```python
from build123d import *

# Parameters (mm, degrees)
F0_R            = 33
F1_DEPTH        = 2.2
F2_R            = 33
F2_R_2          = 30.8
F3_DEPTH        = 12
F4_R            = 2.2
F5_R            = 2.2
F6_R            = 8
F7_DEPTH        = 2.2
F8_R            = 5.75
F9_DEPTH        = 15.3
F10_W           = 1
F10_H           = 63
F11_DEPTH       = 8
F12_W           = 63
F12_H           = 1
F13_DEPTH       = 8
F15_D           = 0.01
F15_DEPTH       = 2.4
F15_CBORE_D     = 12.2
F15_CBORE_DEPTH = 2.4
F15_TIP         = 0.0030043031


with BuildPart() as f1:
    # F0 (on Top) → F1 (new body)
    with BuildSketch(Plane.XY):
        Circle(F0_R)
    extrude(amount=F1_DEPTH)

    # F2 (on face) → F3 (join)
    with BuildSketch(Plane.XY.offset(2.2)):
        Circle(F2_R)
        Circle(F2_R_2, mode=Mode.SUBTRACT)
    extrude(amount=F3_DEPTH)

    # F4
    f4_edges = [f1.edges().sort_by_distance(p)[0] for p in [
        (-33, 0, 0),
    ]]
    fillet(f4_edges, radius=F4_R)

    # F5
    f5_edges = [f1.edges().sort_by_distance(p)[0] for p in [
        (-30.8, 0, 2.2),
    ]]
    fillet(f5_edges, radius=F5_R)

    # F6 (on face) → F7 (join)
    with BuildSketch(Plane.XY.offset(2.2)):
        Circle(F6_R)
    extrude(amount=F7_DEPTH)

    # F8 (on face) → F9 (join)
    with BuildSketch(Plane.XY.offset(4.4)):
        Circle(F8_R)
    extrude(amount=F9_DEPTH)

    # F10 (on face) → F11 (join)
    with BuildSketch(Plane.XY.offset(2.2)):
        Rectangle(F10_W, F10_H)
    extrude(amount=F11_DEPTH)

    # F12 (on face) → F13 (join)
    with BuildSketch(Plane.XY.offset(2.2)):
        Rectangle(F12_W, F12_H)
    extrude(amount=F13_DEPTH)

    # F15
    with Locations(Plane(origin=(0, 0, 0), x_dir=(1, 0, 0), z_dir=(0, 0, -1))):
        with Locations((0, 0)):
            CounterBoreHole(F15_D / 2, F15_CBORE_D / 2, F15_CBORE_DEPTH, depth=F15_DEPTH)
            with Locations((0, 0, -(F15_DEPTH + F15_TIP / 2))):  # 118° drill point
                Cone(0, F15_D / 2, F15_TIP, mode=Mode.SUBTRACT)


solid = f1.part
```
Input: part model. Units: mm. Frame: model coordinates. A direction names the side the tool comes from. Round coordinates to 2 decimals unless told otherwise and drop trailing zeros. Write item = value, one per line.
(1) Material intervals for probe 1 along Y at (x, z) = (0, 11.25); probe 2 along Y at (x, z) = (-6, 7); probe 3 along Z at (x, y) = (-2, -14.5), sorted ascending.
Geometry check:
probe_1 = -33 to -30.8, -5.75 to 5.75, 30.8 to 33
probe_2 = -32.45 to -30.21, -0.5 to 0.5, 30.21 to 32.45
probe_3 = 0 to 2.2
(2) Contact query for flat-ended pins moving along their axis: pin 1 Ø2 at (x, y) = (23, -22) entering from +Z; pin 2 Ø6.5 at (x, z) = (12.5, 4.5) entering from -Y; pin 3 Ø4 at (y, z) = (-18, 7) entering from -X. Output: stop coordinate, or through.
Geometry check:
pin_1 = 14.2
pin_2 = -31.68
pin_3 = -28.86
(3) Access query for faces 1 (the flat face through (-15, 15, 2.2)), 2 (the flat face through (0, 0, 19.7)), 3 (the cylindrical face through (-6.094, -0.268, 1.183)). Directions: +Z, -Z, +X, -X, +Y, -Y. A direction counts if a zero-diameter tool reaches every point of the face in a straight line with its end or side. Return the directions, or none.
Geometry check:
face_1 = +Z
face_2 = +Z, +X, -X, +Y, -Y
face_3 = -Z
